Part model, mm, in its own coordinate system. A direction names the side the tool comes from. Coordinates: 2 decimals unless noted, no trailing zeros. Order: outer loops, then holes, each group sorted by start corner. A loop starts at its lowest first (then second) coordinate and runs counter-clockwise, first axis right, second up. Notation, with made-up numbers: M 4,46 L 19,46 A31 ccw 19,73 Z; hole C 54,-34 d8. An arc over 180 degrees is marked long. Answer in a Markdown table with one row per item. Add a question column.
from build123d import *

# Parameters (mm, degrees)
SKETCH_3_R      = 20
EXTRUDE_3_DEPTH = 50
SKETCH_4_R      = 3
EXTRUDE_4_DEPTH = 5
SKETCH_5_R      = 4
EXTRUDE_5_DEPTH = 10


with BuildPart() as part:
    # 草图3 → 凸台-拉伸3 (new body)
    with BuildSketch(Plane(origin=(0, 0, 0), x_dir=(1, 0, 0), z_dir=(0, 1, 0))):
        with Locations(Location((0, 0, 0), (0, 0, 270))):
            Circle(SKETCH_3_R)
    extrude(amount=EXTRUDE_3_DEPTH)

    # 草图4 → 凸台-拉伸4 (add)
    with BuildSketch(Plane.XZ):
        with Locations(Location((0, 0, 0), (0, 0, 270))):
            Circle(SKETCH_4_R)
    extrude(amount=EXTRUDE_4_DEPTH)

    # 草图5 → 凸台-拉伸5 (add)
    with BuildSketch(Plane(origin=(0, 50, 0), x_dir=(1, 0, 0), z_dir=(0, 1, 0))):
        with Locations(Location((0, 0, 0), (0, 0, 270))):
            Circle(SKETCH_5_R)
    extrude(amount=EXTRUDE_5_DEPTH)


solid = part.part
(1) Slice it at D-D (x = 12.5). List the corners of the cut face in (y, z).
(2) Slice it at A-A (x = 0). List the corners of the cut face in (y, z).
(3) 3-axis set-ups, long thin cutter, end or side, ignore diameter. For faces 1 (the cylindrical face through (-3.905, 54.93, -0.867)), 2 (the flat face through (0, -5, 0)), 3 (the cylindrical face through (0.9, -2.46, -2.86)): which of +Z, -Z, +X, -X, +Y, -Y reach the whole face in a straight line?
(4) Drop flat-ended pins along their axis: P1, Ø3, axis at x = 2, z = -5.5, coming from the -Y side; P2, Ø10, axis at x = 10, z = -10.5, coming from the +Y side; P3, Ø1.5, axis at y = 16.5, z = 7.5, coming from the +X side. Give the stop position or say it passes through.
(5) Slice it at C-C (y = 40.5). List the corners of the cut face in (x, z).
(6) Wall check: line 1 (Y direction, x = 17, z = -6); line 2 (X direction, y = 42.5, z = 14.5); line 3 (X direction, y = 21, z = 13.5). Give the ranges that are in metal, low to high.
(7) Slice it at B-B (z = 0). List the corners of the cut face in (x, y).
Computed:
| question | item | result |
|---|---|---|
| 1 | outline | M 0,-15.61 L 50,-15.61 L 50,15.61 L 0,15.61 Z |
| 2 | outline | M -5,-3 L 0,-3 L 0,-20 L 50,-20 L 50,-4 L 60,-4 L 60,4 L 50,4 L 50,20 L 0,20 L 0,3 L -5,3 Z |
| 3 | face 1 | +Y |
| 3 | face 2 | +Z, -Z, +X, -X, -Y |
| 3 | face 3 | -Y |
| 4 | P1 | stops at y = 0 |
| 4 | P2 | stops at y = 50 |
| 4 | P3 | stops at x = 18.83 |
| 5 | outline | C 0,0 d40 |
| 6 | line 1 | y = 0 to 50 |
| 6 | line 2 | x = -13.77 to 13.77 |
| 6 | line 3 | x = -14.76 to 14.76 |
| 7 | outline | M -20,0 L -3,0 L -3,-5 L 3,-5 L 3,0 L 20,0 L 20,50 L 4,50 L 4,60 L -4,60 L -4,50 L -20,50 Z |
